For this review, take the finished solid that the model builds, in its own axes (mm). A direction names the side the tool comes from. Coordinates: 2 decimals unless noted, no trailing zeros. Loops run counter-clockwise (first coordinate to the right, second up) from the corner with the lowest first, then second, coordinate; pieces in that order, holes last. Notation, with made-up numbers: (37, 15.5) -> (71, 15.5) arc R12 ccw to (71, 27.5) -> close; hole circle Ø7 at (-30.75, -22.75). An arc over 180 degrees is marked (long way). One line per item, written item: value.
from build123d import *

# Parameters (mm, degrees)
CROQUIS1_R              = 5.5
CROQUIS1_R_2            = 2
SALIENTE_EXTRUIR1_DEPTH = 10
CROQUIS2_R              = 8
CROQUIS2_R_2            = 2
SALIENTE_EXTRUIR3_DEPTH = 1.5
SALIENTE_EXTRUIR5_START = 8.5
CROQUIS2_3_R            = 8
CROQUIS2_3_R_2          = 2
SALIENTE_EXTRUIR5_DEPTH = 1.5
CHAFL_N1_SIZE           = 0.1


with BuildPart() as part:
    # Croquis1 → Saliente-Extruir1 (new body)
    with BuildSketch(Plane.XY):
        Circle(CROQUIS1_R)
        Circle(CROQUIS1_R_2, mode=Mode.SUBTRACT)
    extrude(amount=SALIENTE_EXTRUIR1_DEPTH)

    # Croquis2 → Saliente-Extruir3 (add)
    with BuildSketch(Plane.XY):
        Circle(CROQUIS2_R)
        Circle(CROQUIS2_R_2, mode=Mode.SUBTRACT)
    extrude(amount=SALIENTE_EXTRUIR3_DEPTH)

    # Croquis2<3> → Saliente-Extruir5 (add)
    with BuildSketch(Plane.XY.offset(SALIENTE_EXTRUIR5_START)):
        Circle(CROQUIS2_3_R)
        Circle(CROQUIS2_3_R_2, mode=Mode.SUBTRACT)
    extrude(amount=SALIENTE_EXTRUIR5_DEPTH)

    # Chaflán1
    chafl_n1_edges = [part.edges().sort_by_distance(p)[0] for p in [
        (-8, 0, 1.5),
        (-8, 0, 0),
        (-8, 0, 10),
        (-8, 0, 8.5),
    ]]
    chamfer(chafl_n1_edges, length=CHAFL_N1_SIZE)

    # Croquis3 → Cortar-Revolución1 (revolve, cut)
    with BuildSketch(Plane(origin=(0, 0, 0), x_dir=(1, 0, 0), z_dir=(0, 1, 0))):
        with BuildLine():
            Line((-2, 0), (-2.05, -0.1))
            Line((-2.05, -0.1), (-2.1, 0))
            Line((-2.1, 0), (-2.5, 0))
            ThreePointArc((-2.5, 0), (-3, -0.210102051), (-3.5, 0))
            Line((-3.5, 0), (-3.9, 0))
            Line((-3.9, 0), (-3.95, -0.1))
            Line((-3.95, -0.1), (-4, 0))
            Line((-4, 0), (-4, 0.1))
            Line((-4, 0.1), (-2, 0.1))
            Line((-2, 0.1), (-2, 0))
        make_face()
        with BuildLine():
            Line((-2, -10.1), (-2, -10))
            Line((-2, -10), (-2.05, -9.9))
            Line((-2.05, -9.9), (-2.1, -10))
            Line((-2.1, -10), (-2.5, -10))
            ThreePointArc((-2.5, -10), (-3, -9.789897949), (-3.5, -10))
            Line((-3.5, -10), (-3.9, -10))
            Line((-3.9, -10), (-3.95, -9.9))
            Line((-3.95, -9.9), (-4, -10))
            Line((-4, -10), (-4, -10.1))
            Line((-4, -10.1), (-2, -10.1))
        make_face()
    revolve(axis=Axis((0, 0, 0), (0, 0, 1)), mode=Mode.SUBTRACT)


solid = part.part
1. For faces 1 (the cylindrical face through (-1.73, -7.81, 9.24)), 2 (the cylindrical face through (-1.19, -5.37, 4.95)), list the 3-axis set-ups (+Z, -Z, +X, -X, +Y, -Y) from which the entire face can be reached by the end or side of a thin tool; tool diameter is ignored.
Return value:
face 1: +Z, -Z
face 2: none
2. Take a section at A-A, the plane z = 6.75. Give the boundary of the cut face in (x, y), and give its area (3 significant figures).
Return value:
outline: circle Ø11 at (0, 0); hole circle Ø4 at (0, 0)
area: 82.5 mm2
3. To check wall thickness, follow probe 1 along Y at (x, z) = (0, 2.5); probe 2 along Z at (x, y) = (2.25, 6.25). State the ranges of each line that lie inside material, in increasing order. Write a range as from..to.
Return value:
probe 1: y = -5.5..-2, 2..5.5
probe 2: z = 0..1.5, 8.5..10
4. Insertion check: pin 1 Ø3 at (y, z) = (4.5, 5.5) entering from -X; pin 2 Ø3 at (y, z) = (1.5, 8) entering from -X. Each pin has a flat end and moves straight along its axis. Give the tip position at first contact, or say it passes through.
Return value:
pin 1: stops at x = -4.61
pin 2: stops at x = -8
5. The part is to be moulded in two halves that separate along X. For faces 3 (the cylindrical face through (-1.73, -7.81, 0.74)), 4 (the cylindrical face through (0, -2, 5)), 5 (the flat face through (-1.9, 5.4, 1.5)), say which applies: pulls with the +X half, pulls with the -X half, needs draft (parallel to the pull), parting line crosses it, or undercut.
Return value:
face 3: parting line crosses it
face 4: undercut
face 5: needs draft
